from build123d import *

# Parameters (mm, degrees)
SKETCH1_W           = 60
SKETCH1_H           = 30
BOSS_EXTRUDE1_DEPTH = 5
SKETCH2_R           = 6.41363938
SKETCH2_R_2         = 3.302926723
BOSS_EXTRUDE2_DEPTH = 20
SKETCH3_R           = 6.356146431
SKETCH3_R_2         = 3.302926723
BOSS_EXTRUDE3_DEPTH = 20


with BuildPart() as part:
    # Sketch1 → Boss-Extrude1 (new body)
    with BuildSketch(Plane.XY):
        with Locations((30, -15)):
            Rectangle(SKETCH1_W, SKETCH1_H)
    extrude(amount=BOSS_EXTRUDE1_DEPTH)

    # Sketch2 → Boss-Extrude2 (add)
    with BuildSketch(Plane(origin=(60, 0, 0), x_dir=(0, 0, -1), z_dir=(1, 0, 0))):
        with Locations((0, 3.924359496)):
            Circle(SKETCH2_R)
        with Locations((0, 3.924359496)):
            Circle(SKETCH2_R_2, mode=Mode.SUBTRACT)
    extrude(amount=-BOSS_EXTRUDE2_DEPTH)

    # Sketch3 → Boss-Extrude3 (add)
    with BuildSketch(Plane.ZY):
        with Locations((0, 3.924359496)):
            Circle(SKETCH3_R)
        with Locations((0, 3.924359496)):
            Circle(SKETCH3_R_2, mode=Mode.SUBTRACT)
    extrude(amount=-BOSS_EXTRUDE3_DEPTH)


solid = part.part
Read the model definition and answer for the solid it produces. Units are mm, in the model's axes. A direction names the side the tool comes from. Round coordinates to 2 decimals unless told otherwise and drop trailing zeros. Loops run counter-clockwise (first coordinate to the right, second up) from the corner with the lowest first, then second, coordinate; pieces in that order, holes last.
Q1. Determine the mould class of faces 6 (the face through (50.14, 9.6, -2.99)), 7 (the face through (50.14, 0.7, 0.72)), 8 (the face through (9.86, 0.7, -0.72)), 9 (the face through (30, 0, 2)) for opening direction Z: released by +Z, released by -Z, zero draft, split by the parting line, or undercut.
Q2. Section C-C on z = -4.5 is taken. Write down the section's boundary in (x, y), and give its area (3 significant figures).
Q3. Which of the six approach directions +Z, -Z, +X, -X, +Y, -Y give full straight-line access (tool end or side, diameter ignored) to faces 1 (the face through (20, 7, -3)), 2 (the face through (60, -10, 2)), 3 (the face through (0, -5, 1)), 4 (the face through (9.86, 9.74, -2.56)), 5 (the face through (30, -15, 5))?
Q4. Section A-A on y = 6 is taken. Write down the section's boundary in (x, z), and give its area (3 significant figures).
Q5. Section D-D on x = 19 is taken. Write down the section's boundary in (y, z).
Q6. Each of these flat-tipped pins is pushed along its axis until it touches: pin 1 (9 mm diameter, centred on x = 35, y = -15, fed in from +Z); pin 2 (5.5 mm diameter, centred on x = 30.5, z = 2.5, fed in from +Y); pin 3 (4 mm diameter, centred on x = 48, y = 5.5, fed in from -Z); pin 4 (1 mm diameter, centred on x = 15, y = -2, fed in from -Z). Where does it stop, or does it pass through?
Q7. Section B-B on z = -1.5 is taken. Write down the section's boundary in (x, y), and give its area (3 significant figures).
Q8. Consider probe 1 along Z at (x, y) = (34.5, -2); probe 2 along Z at (x, y) = (19, 3); probe 3 along Z at (x, y) = (11.5, 5). Determine where each line is inside the solid, lowest interval first.
Output:
1. face 6: split by the parting line
1. face 7: undercut
1. face 8: undercut
1. face 9: zero draft
2. outline: (0, -0.56) - (20, -0.56) - (20, 8.41) - (0, 8.41) - close; (40, -0.65) - (60, -0.65) - (60, 8.49) - (40, 8.49) - close
2. area: 362 mm2
3. face 1: -Z, +Y
3. face 2: +Z, -Z, +X, +Y, -Y
3. face 3: +Z, -Z, -X, +Y, -Y
3. face 4: -X
3. face 5: +Z, +X, -X, -Y
4. outline: (0, -6.01) - (20, -6.01) - (20, -2.57) - (0, -2.57) - close; (0, 2.57) - (20, 2.57) - (20, 6.01) - (0, 6.01) - close; (40, -6.07) - (60, -6.07) - (60, -2.57) - (40, -2.57) - close; (40, 2.57) - (60, 2.57) - (60, 6.07) - (40, 6.07) - close
4. area: 278 mm2
5. outline: (-30, 0) - (-2.43, 0) arc R6.36 ccw (long way) to (0, 5) - (-30, 5) - close; hole circle Ø6.61 at (3.92, 0)
6. pin 1: stops at z = 5
6. pin 2: stops at y = 0
6. pin 3: stops at z = -6.41
6. pin 4: stops at z = -3.31
7. outline: (0, -2.25) - (20, -2.25) - (20, 0.98) - (0, 0.98) - close; (0, 6.87) - (20, 6.87) - (20, 10.1) - (0, 10.1) - close; (40, -2.31) - (60, -2.31) - (60, 0.98) - (40, 0.98) - close; (40, 6.87) - (60, 6.87) - (60, 10.16) - (40, 10.16) - close
7. area: 261 mm2
8. probe 1: z = 0 to 5
8. probe 2: z = -6.29 to -3.17, 3.17 to 6.29
8. probe 3: z = -6.26 to -3.12, 3.12 to 6.26
